Autodesk Inventor part; units mm, degrees
ref_plane "Work Plane1" through (2, 0, -1.905) normal (0, 0, -1) x (-1, 0, 0)
ref_plane "YZ Plane" through (0, 0, 0) normal (1, 0, 0) x (0, 1, 0)
ref_plane "XZ Plane" through (0, 0, 0) normal (0, 1, 0) x (-1, 0, 0)
sketch "Sketch1" plane through (0, 0, 0) normal (0, 1, 0) x (-1, 0, 0)
  line L0 (2, 2.5) -> (-2, 2.5)
  line L1 (-2, 2.5) -> (-2, -2.5)
  line L2 (-2, -2.5) -> (2, -2.5)
  line L3 (2, -2.5) -> (2, 2.5)
  point P0 (0, 0)
  dimension "d0" = 4
  dimension "d1" = 5
  dimension "d2" = 2
  dimension "d3" = 2.5
extrude "Extrusion1" add sketch "Sketch1" along normal blind 1.65
chamfer "Chamfer1" distance 0.5 angle 10 1 edges at (0, 1.65, 2.5) measured on face at (-0.6667, 0.55, 2.5)
chamfer "Chamfer2" distance 0.5 angle 10 1 edges at (-2, 1.65, -0.0441) measured on face at (-2, 0.9333, -0.8333)
chamfer "Chamfer3" distance 0.5 angle 10 1 edges at (0.0441, 1.65, -2.5) measured on face at (0.6667, 0.9333, -2.5)
chamfer "Chamfer4" distance 0.5 angle 45 1 edges at (2, 1.65, 0) measured on face at (2, 0.3833, 0.8333)
ref_plane "Work Plane1" through (2, 0, -1.905) normal (0, 0, -1) x (-1, 0, 0)
sketch "Sketch2" plane through (2, 0, -1.905) normal (0, 0, -1) x (-1, 0, 0)
  line L0 (0, 0.825) -> (0, 0.575)
  line L1 (0, 0.575) -> (-0.3809, 0.575)
  line L2 (-0.3809, 0.575) -> (-0.7, -0.25)
  line L3 (-0.7, -0.25) -> (-1.1, -0.25)
  line L4 (-1.1, -0.25) -> (-1.1, 0)
  line L5 (-1.1, 0) -> (-0.8681, 0)
  line L6 (-0.8681, 0) -> (-0.549, 0.825)
  line L7 (-0.549, 0.825) -> (0, 0.825)
  line L8 (0, 0) -> (0, 1.15)
  line L9 (0, 0) -> (4, 0)
  point P0 (2, 0)
  dimension "d19" = 0
  dimension "d20" = 0.25
  dimension "d21" = 0.25
  dimension "d22" = 0.4
  dimension "d23" = 1.1
  dimension "d24" = 0.25
  dimension "d25" = 0.825
extrude "Extrusion2" add sketch "Sketch2" along normal mid plane 0.51
pattern_linear "Rectangular Pattern1" count 4 spacing 1.27 along (0, 0, 1) of "Extrusion2"
mirror "Mirror1" about plane through (0, 0, 0) normal (1, 0, 0) of "Extrusion2", "Rectangular Pattern1"
properties part number "MC34063"
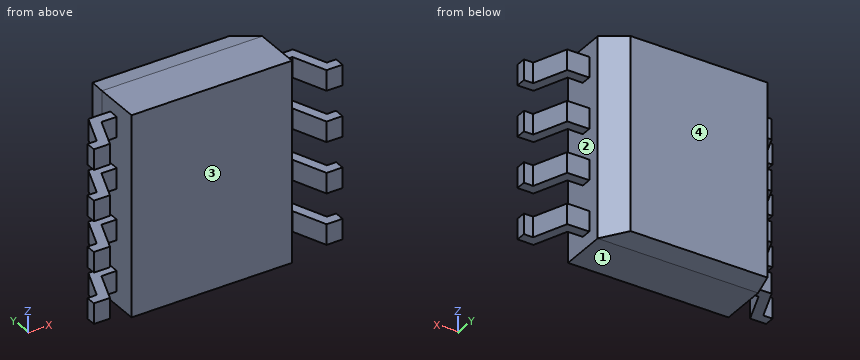
Input: part model. Units: mm. Frame: model coordinates. Face numbers are marked on the shaded views. A direction names the side the tool comes from. Round coordinates to 2 decimals unless told otherwise and drop trailing zeros. Loops run counter-clockwise (first coordinate to the right, second up) from the corner with the lowest first, then second, coordinate; pieces in that order, holes last. Notation, with made-up numbers: M -35,27 L -6,27 A28 cw -6,53 Z; hole C -1.5,25.25 d10. An arc over 180 degrees is marked long. Answer in a Markdown table with one row per item. Add a question column.
1. Mould query, pull axis X, two halves, no side actions, for the marked faces 1 and 2. Classes: released by +X, released by -X, zero draft, split by the parting line, or undercut.
2. Section A-A (z = -1). Output: boundary loops of the cut face in (x, y).
3. Ray query, probe 1 along X at (y, z) = (0.4, -1.85); probe 2 along Y at (x, z) = (-0.25, -2.2); probe 3 along X at (y, z) = (0.05, 1.1). Return the intervals inside material, ascending.
4. Section C-C (y = 0.9). Output: boundary loops of the cut face in (x, z), and give its area (3 significant figures).
5. Contact query for flat-ended pins moving along their axis: pin 1 (0.9 mm diameter, centred on x = -2.5, y = 0.5, fed in from +Z); pin 2 (0.9 mm diameter, centred on x = -2.5, y = 0.5, fed in from -Z); pin 3 (0.6 mm diameter, centred on x = 2.5, z = 2, fed in from +Y) (3 decimals). Output: stop coordinate, or through.
6. Section B-B (x = 0.5). Output: boundary loops of the cut face in (y, z), and give its area (3 significant figures).
7. Set-up query: the marked faces 3 and 4. Return all of +Z, -Z, +X, -X, +Y, -Y with unobstructed straight access to the full face (end or side cutting, diameter ignored); none if empty.
8. Section D-D (y = 1.5). Output: boundary loops of the cut face in (x, z).
Values follow:
| question | item | result |
|---|---|---|
| 1 | face 1 | zero draft |
| 1 | face 2 | undercut |
| 2 | outline | M -2,0 L 2,0 L 2,1.15 L 1.5,1.65 L -1.91,1.65 L -2,1.15 Z |
| 3 | probe 1 | -2.71 to -2.45, -2 to 2, 2.45 to 2.71 |
| 3 | probe 2 | 0 to 1.65 |
| 3 | probe 3 | -2 to 2 |
| 4 | outline | M -2,-2.5 L 2,-2.5 L 2,2.5 L -2,2.5 Z |
| 4 | area | 20.0 mm^2 |
| 5 | pin 1 | z = 2.16 |
| 5 | pin 2 | z = -2.16 |
| 5 | pin 3 | y = 0.825 |
| 6 | outline | M 0,-2.5 L 1.15,-2.5 L 1.65,-2.41 L 1.65,2.41 L 1.15,2.5 L 0,2.5 Z |
| 6 | area | 8.21 mm^2 |
| 7 | face 3 | +Z, -Z, -Y |
| 7 | face 4 | +Z, -Z, +X, -X, +Y |
| 8 | outline | M -1.94,-2.44 L 1.65,-2.44 L 1.65,2.44 L -1.94,2.44 Z |
